```python
from build123d import *

# Parameters (mm, degrees)
ESQUISSE1_R                = 38.1
BOSS_EXTRU_1_DEPTH         = 25.5
ESQUISSE3_R                = 25.4
ENL_V_MAT_EXTRU_2_DEPTH    = 20.5
ESQUISSE5_R                = 11
ENL_V_MAT_EXTRU_3_DEPTH    = 5
ESQUISSE7_R                = 12.7
ENL_V_MAT_EXTRU_4_DEPTH    = 1
ESQUISSE8_R                = 38.1
ESQUISSE8_R_2              = 34.925
ENL_V_MAT_EXTRU_5_DEPTH    = 2
R_P_TITION_LIN_AIRE1_COUNT = 6
R_P_TITION_LIN_AIRE1_PITCH = 4
ESQUISSE9_R                = 2.5
ENL_V_MAT_EXTRU_6_DEPTH    = 26.5


with BuildPart() as part:
    # Esquisse1 → Boss.-Extru.1 (new body)
    with BuildSketch(Plane.XY):
        with Locations((23.679503876, 29.670703652)):
            Circle(ESQUISSE1_R)
    extrude(amount=BOSS_EXTRU_1_DEPTH)

    # Esquisse3 → Enlèv. mat.-Extru.2 (cut)
    with BuildSketch(Plane.XY.offset(25.5)):
        with Locations((23.679503876, 29.670703652)):
            Circle(ESQUISSE3_R)
    extrude(amount=-ENL_V_MAT_EXTRU_2_DEPTH, mode=Mode.SUBTRACT)

    # Esquisse5 → Enlèv. mat.-Extru.3 (cut)
    with BuildSketch(Plane(origin=(0, 0, 0), x_dir=(-1, 0, 0), z_dir=(0, 0, -1))):
        with Locations((-23.679503876, 29.670703652)):
            Circle(ESQUISSE5_R)
    extrude(amount=-ENL_V_MAT_EXTRU_3_DEPTH, mode=Mode.SUBTRACT)

    # Esquisse7 → Enlèv. mat.-Extru.4 (cut)
    with BuildSketch(Plane(origin=(0, 0, 0), x_dir=(-1, 0, 0), z_dir=(0, 0, -1))):
        with Locations((-23.679503876, 29.670703652)):
            Circle(ESQUISSE7_R)
    extrude(amount=-ENL_V_MAT_EXTRU_4_DEPTH, mode=Mode.SUBTRACT)

    # Esquisse8 → Enlèv. mat.-Extru.5 (cut)
    with BuildSketch(Plane.XY.offset(25.5)):
        with Locations((23.679503876, 29.670703652)):
            Circle(ESQUISSE8_R)
        with Locations((23.679503876, 29.670703652)):
            Circle(ESQUISSE8_R_2, mode=Mode.SUBTRACT)
    enl_v_mat_extru_5 = extrude(amount=-ENL_V_MAT_EXTRU_5_DEPTH, mode=Mode.SUBTRACT)

    # Répétition linéaire1: Enlèv. mat.-Extru.5 ×6
    with Locations(*[(0, 0, -i * R_P_TITION_LIN_AIRE1_PITCH) for i in range(1, R_P_TITION_LIN_AIRE1_COUNT)]):
        add(enl_v_mat_extru_5, mode=Mode.SUBTRACT)

    # Esquisse9 → Enlèv. mat.-Extru.6 (cut, through all)
    with BuildSketch(Plane(origin=(0, 0, 0), x_dir=(-1, 0, 0), z_dir=(0, 0, -1))):
        with Locations((6.482996124, 29.670703652)):
            Circle(ESQUISSE9_R)
        with Locations((-53.842003876, 29.670703652)):
            Circle(ESQUISSE9_R)
    extrude(amount=-ENL_V_MAT_EXTRU_6_DEPTH, mode=Mode.SUBTRACT)


solid = part.part
```
Source: CAD feature listing. Evaluate the final solid. Frame: model axes, mm. A direction names the side the tool comes from. Round coordinates to 2 decimals unless told otherwise and drop trailing zeros. Loops run counter-clockwise (first coordinate to the right, second up) from the corner with the lowest first, then second, coordinate; pieces in that order, holes last. Notation, with made-up numbers: M 29,57.25 L 71,57.25 A7 ccw 71,63.25 Z; hole C -13,40.25 d4. An arc over 180 degrees is marked long. Put each result on its own line as item: value.
(1) Pull-direction query (Y, two-part tool) for faces 1 (the face through (56.992, 40.161, 16.514)), 2 (the face through (40.4, -1.2, 21.5)), 3 (the face through (-7.637, 27.453, 12.572)); classes: released by +Y, released by -Y, zero draft, split by the parting line, or undercut.
Solutions:
face 1: split by the parting line
face 2: zero draft
face 3: undercut
(2) First-contact query: pin 1 (5 mm diameter, centred on x = 34.5, z = 14, fed in from -Y); pin 2 (1.5 mm diameter, centred on x = 13.5, z = 16.5, fed in from +Y); pin 3 (1.5 mm diameter, centred on y = 38, z = 10.5, fed in from +X). Flat tips, straight axial feed; report the tip coordinate or a pass-through.
Solutions:
pin 1: y = -7.51
pin 2: y = 63.3
pin 3: x = 61.02
(3) Section A-A, the plane z = 6.5. Return loops of the section in (x, y), and give its area (3 significant figures).
Solutions:
outline: C 23.68,29.67 d76.2; hole C -6.48,29.67 d5; hole C 23.68,29.67 d50.8; hole C 53.84,29.67 d5
area: 2,490 mm²
(4) Access query for faces 4 (the face through (40.4, -1.2, 19.5)), 5 (the face through (28, 40, 1)), 6 (the face through (13, 53, 25.5)), 7 (the face through (15.42, -7.523, 1.726)), 8 (the face through (56.992, 40.161, 24.514)). Directions: +Z, -Z, +X, -X, +Y, -Y. A direction counts if a zero-diameter tool reaches every point of the face in a straight line with its end or side. Return the directions, or none.
Solutions:
face 4: none
face 5: -Z
face 6: +Z, +X, -X, +Y, -Y
face 7: +Z, -Z
face 8: +Z
(5) Ray query, line 1 (Z direction, x = 11.5, y = 65); line 2 (X direction, y = 30, z = 2.75); line 3 (X direction, y = 29, z = 13.25). Return the intervals inside material, ascending. Write a range as [from, to].
Solutions:
line 1: [0, 3.5], [5.5, 7.5], [9.5, 11.5], [13.5, 15.5], [17.5, 19.5], [21.5, 23.5]
line 2: [-14.42, -8.96], [-4, 12.68], [34.67, 51.36], [56.32, 61.78]
line 3: [-11.24, -8.89], [-4.07, -1.71], [49.07, 51.43], [56.25, 58.6]
